Here's the drawing with two shaded views (mm, measured from the low corner). I have some questions. A direction names the side the tool comes from. Coordinates: 2 decimals unless noted, no trailing zeros. Order: outer loops, then holes, each group sorted by start corner. A loop starts at its lowest first (then second) coordinate and runs counter-clockwise, first axis right, second up. Notation, with made-up numbers: (32, 65.25) - (61, 65.25) arc R30 ccw to (61, 90.25) - close; hole circle Ø3 at (57.5, -13.75). An arc over 180 degrees is marked (long way). One line per item, written item: value. Start each with the question number.
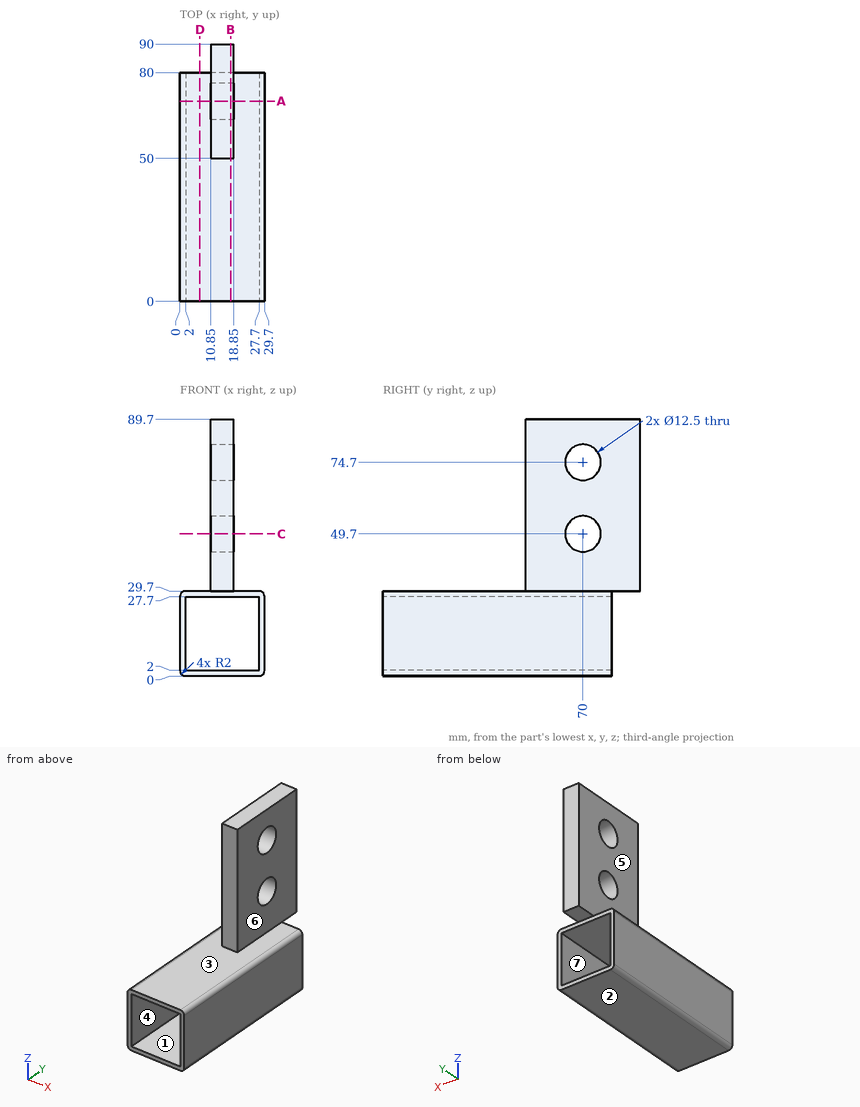
Q1. Which directions (+Z, -Z, +X, -X, +Y, -Y) give clear straight access to the entire face, cutting with the end or side of a thin tool? Please do the marked faces 1, 2 and 3.
Q2. I want a section at A-A on y = 70. Please give me the cut outline in (x, z), then the cut area to 3 significant figures.
Q3. We'd pull the mould along X, two halves only. Please class the marked faces 4, 5, 6 and 7: +X half, -X half, draft (parallel to the pull), parting line (faces both ways), or undercut.
Q4. I want a section at B-B on x = 17.75. Please give me the cut outline in (y, z).
Q5. I'm going to push flat-ended pins straight in: pin 1 (15 mm diameter, centred on x = 11, z = 8, fed in from +Y); pin 2 (5 mm diameter, centred on y = 67.5, z = 41.5, fed in from -X); pin 3 (13 mm diameter, centred on x = 11.5, y = 40, fed in from +Z); pin 4 (11 mm diameter, centred on y = 70, z = 49.7, fed in from -X). Where does each tip first touch, or does it pass through?
Q6. I want a section at C-C on z = 49.7. Please give me the cut outline in (x, y).
Q7. If I drill on L1, parallel to Z at x = 16.25, y = 70; L2, parallel to X at y = 39.5, z = 24.5, over which ranges is the centre line in solid material (lowest first)?
Q8. I want a section at D-D on x = 7. Please give me the cut outline in (y, z), then the cut area to 3 significant figures.
Values follow:
1. face 1: +Y, -Y
1. face 2: -Z, +X, -X, +Y, -Y
1. face 3: +Z, -Y
2. outline: (0, 2) arc R2 ccw to (2, 0) - (27.7, 0) arc R2 ccw to (29.7, 2) - (29.7, 27.7) arc R2 ccw to (27.7, 29.7) - (18.85, 29.7) - (18.85, 43.45) - (10.85, 43.45) - (10.85, 29.7) - (2, 29.7) arc R2 ccw to (0, 27.7) - close; (10.85, 55.95) - (18.85, 55.95) - (18.85, 68.45) - (10.85, 68.45) - close; (10.85, 80.95) - (18.85, 80.95) - (18.85, 89.7) - (10.85, 89.7) - close; hole (2, 2) - (27.7, 2) - (27.7, 27.7) - (2, 27.7) - close
2. area: 498 mm^2
3. face 4: undercut
3. face 5: -X half
3. face 6: +X half
3. face 7: undercut
4. outline: (0, 0) - (80, 0) - (80, 2) - (0, 2) - close; (0, 27.7) - (80, 27.7) - (80, 29.7) - (90, 29.7) - (90, 89.7) - (50, 89.7) - (50, 29.7) - (0, 29.7) - close; hole circle Ø12.5 at (70, 49.7); hole circle Ø12.5 at (70, 74.7)
5. pin 1: stops at y = 80
5. pin 2: stops at x = 10.85
5. pin 3: stops at z = 29.7
5. pin 4: passes through
6. outline: (10.85, 50) - (18.85, 50) - (18.85, 63.75) - (10.85, 63.75) - close; (10.85, 76.25) - (18.85, 76.25) - (18.85, 90) - (10.85, 90) - close
7. L1: z = 0 to 2, 27.7 to 43.45, 55.95 to 68.45, 80.95 to 89.7
7. L2: x = 0 to 2, 27.7 to 29.7
8. outline: (0, 0) - (80, 0) - (80, 2) - (0, 2) - close; (0, 27.7) - (80, 27.7) - (80, 29.7) - (0, 29.7) - close
8. area: 320 mm^2
